Autodesk Inventor part; units mm, degrees
ref_plane "工作平面1" through (0, 6, 0) normal (0, 1, 0) x (1, 0, 0)
ref_plane "YZ Plane" through (0, 0, 0) normal (1, 0, 0) x (0, 1, 0)
ref_plane "XZ Plane" through (0, 0, 0) normal (0, 1, 0) x (-1, 0, 0)
sketch "草图1" plane through (0, 0, 0) normal (0, 1, 0) x (-1, 0, 0)
  circle A0 centre (0, 0) radius 5
  dimension "d0" = 10
extrude "拉伸1" add sketch "草图1" along normal blind 1
sketch "草图2" plane through (0, 1, 0) normal (0, 1, 0) x (1, 0, 0)
  circle A0 centre (0, 0) radius 4
  dimension "d3" = 8
ref_plane "工作平面1" through (0, 6, 0) normal (0, 1, 0) x (1, 0, 0)
sketch "草图3" plane through (0, 6, 0) normal (0, 1, 0) x (1, 0, 0)
  circle A0 centre (0, 0) radius 4.5
  dimension "d5" = 9
loft "放样1" add profiles "草图2", "草图3"
sketch "草图4" plane through (0, 0, 0) normal (0, -1, 0) x (1, 0, 0)
  circle A0 centre (0, 0) radius 4
  dimension "d11" = 8
extrude "拉伸2" add sketch "草图4" along normal blind 5
properties part number "backtop"
Here's how the part is built. I have some questions about the finished solid (model axes, mm). Coordinates: 2 decimals unless noted, no trailing zeros. Loops run counter-clockwise (first coordinate to the right, second up) from the corner with the lowest first, then second, coordinate; pieces in that order, holes last.
1. Imagine slicing it at A-A, the plane x = 0. Please give me the cut outline in (y, z).
2. For P1, Ø2, axis at y = 4, z = -3, coming from the -X side; P2, Ø3, axis at x = -2.5, y = -3.5, coming from the +Z side; P3, Ø3, axis at x = 0.5, y = 3.5, coming from the +Z side, each with a flat end and sliding along its axis, tell me the tip position at first contact or that it passes through.
3. If we mould it in two halves opening along Y, with no side actions, what happens to faces 1 (the cylindrical face through (-0.867, -2.465, 3.905)), 2 (the flat face through (0, -5, 0)), 3 (the conical face through (2.26, 2.98, -3.54))? For each: pulls with the +Y half, pulls with the -Y half, needs draft (parallel to the pull), parting line crosses it, or undercut.
4. I need wall thicknesses on L1, parallel to Z at x = 1, y = -4; L2, parallel to Z at x = 2, y = 5.5; L3, parallel to X at y = -0.5, z = 3.5. Which ranges of each line are inside material? Lowest first, please.
5. Imagine slicing it at B-B, the plane y = 1.5. Please give me the cut outline in (x, z).
6. Imagine slicing it at C-C, the plane y = 0.25. Please give me the cut outline in (x, z), and give its area (3 significant figures).
Taken from the geometry:
1. outline: (-5, -4) - (0, -4) - (0, -5) - (1, -5) - (1, -4) - (6, -4.5) - (6, 4.5) - (1, 4) - (1, 5) - (0, 5) - (0, 4) - (-5, 4) - close
2. P1: stops at x = -3.82
2. P2: stops at z = 3.87
2. P3: stops at z = 4.39
3. face 1: needs draft
3. face 2: pulls with the -Y half
3. face 3: undercut
4. L1: z = -3.87 to 3.87
4. L2: z = -3.98 to 3.98
4. L3: x = -1.94 to 1.94
5. outline: circle Ø8.1 at (0, 0)
6. outline: circle Ø10 at (0, 0)
6. area: 78.5 mm2
